```python
from build123d import *

# Parameters (mm, degrees)
RACCORDO1_R              = 1
SMUSSO1_SIZE             = 1
RACCORDO2_R              = 1
TAGLIO_ESTRUSIONE1_DEPTH = 36.80502758


with BuildPart() as part:
    # Schizzo1 → Rivoluzione1 (revolve)
    with BuildSketch(Plane.XY, mode=Mode.PRIVATE) as rivoluzione1_sk:
        Polygon((10.5, 7), (21, 7), (21, 1), (10, 1), (10, 0), (6, 0), (6, 27), (9.5, 27), (9.5, 12), (10.5, 12), align=None)
    revolve(rivoluzione1_sk.sketch.rotate(Axis((0, 27, 0), (0, -1, 0)), 90), axis=Axis((0, 27, 0), (0, -1, 0)))

    # Raccordo1
    raccordo1_edges = [part.edges().sort_by_distance(p)[0] for p in [
        (0, 12, -9.5),
    ]]
    fillet(raccordo1_edges, radius=RACCORDO1_R - 0.0001)  # a hair under: the kernel refuses the full size

    # Smusso1
    smusso1_edges = [part.edges().sort_by_distance(p)[0] for p in [
        (0, 27, -9.5),
    ]]
    chamfer(smusso1_edges, length=SMUSSO1_SIZE)

    # Raccordo2
    raccordo2_edges = [part.edges().sort_by_distance(p)[0] for p in [
        (0, 1, -10),
    ]]
    fillet(raccordo2_edges, radius=RACCORDO2_R - 0.0001)  # a hair under: the kernel refuses the full size

    # Schizzo2 → Taglio-Estrusione1 (cut, through all)
    with BuildSketch(Plane(origin=(0, 7, 0), x_dir=(1, 0, 0), z_dir=(0, 1, 0))):
        with BuildLine():
            ThreePointArc((2.25, 15.5), (1.590990258, 17.090990258), (0, 17.75))
            Line((0, 17.75), (0, 13.25))
            ThreePointArc((0, 13.25), (1.590990258, 13.909009742), (2.25, 15.5))
        make_face()
        with BuildLine():
            Line((0, 13.25), (0, 17.75))
            ThreePointArc((0, 17.75), (-2.25, 15.5), (0, 13.25))
        make_face()
        with BuildLine():
            ThreePointArc((17.75, 0), (15.5, 2.25), (13.25, 0))
            Line((13.25, 0), (17.75, 0))
        make_face()
        with BuildLine():
            Line((17.75, 0), (13.25, 0))
            ThreePointArc((13.25, 0), (15.5, -2.25), (17.75, 0))
        make_face()
        with BuildLine():
            ThreePointArc((2.25, -15.5), (1.590990258, -13.909009742), (0, -13.25))
            Line((0, -13.25), (0, -17.75))
            ThreePointArc((0, -17.75), (1.590990258, -17.090990258), (2.25, -15.5))
        make_face()
        with BuildLine():
            Line((0, -17.75), (0, -13.25))
            ThreePointArc((0, -13.25), (-2.25, -15.5), (0, -17.75))
        make_face()
        with BuildLine():
            ThreePointArc((-17.75, 0), (-15.5, -2.25), (-13.25, 0))
            Line((-13.25, 0), (-17.75, 0))
        make_face()
        with BuildLine():
            Line((-17.75, 0), (-13.25, 0))
            ThreePointArc((-13.25, 0), (-15.5, 2.25), (-17.75, 0))
        make_face()
    extrude(amount=-TAGLIO_ESTRUSIONE1_DEPTH, mode=Mode.SUBTRACT)


solid = part.part
```
Work out the finished part from the listing and answer in its coordinate system (mm). A direction names the side the tool comes from. Give positions to 0.01 mm unless a question says otherwise; leave off trailing zeros. Loops run counter-clockwise (first coordinate to the right, second up) from the corner with the lowest first, then second, coordinate; pieces in that order, holes last. Notation, with made-up numbers: (-36.75, 72) - (-20.75, 72) arc R5 cw to (-20.75, 79) - close; hole circle Ø10 at (-11.5, -36.75). An arc over 180 degrees is marked (long way). One line per question, with ' | ' between items.
(1) A tool of negligible diameter and unlimited length cuts with its end or side. For faces 1 (the face through (-6, 27, -2)), 2 (the face through (-3.2, 9.5, 10)), 3 (the face through (9, 1, 9)), from which of +Z, -Z, +X, -X, +Y, -Y can it reach the whole face along a straight path? Write none if from no direction.
Recorded:
face 1: +Z, -Z, +X, -X, +Y | face 2: +Y | face 3: -Y
(2) The part is cut by section C-C (x = -16). Write down the section's boundary in (y, z).
Recorded:
outline: (1, -13.6) - (7, -13.6) - (7, -2.19) - (1, -2.19) - close; (1, 2.19) - (7, 2.19) - (7, 13.6) - (1, 13.6) - close
(3) The mould has two halves that part along Z. Classify faces 4 (the face through (-1.802, 13.689, 5.723)), 5 (the face through (-10, 7, -4)), 6 (the face through (-6.31, 3.96, 20.03)): +Z half, -Z half, draft (parallel to the pull), parting line (faces both ways), or undercut.
Recorded:
face 4: undercut | face 5: draft | face 6: parting line
(4) Straight lines are drawn through the part: probe 1 along X at (y, z) = (11.75, 0); probe 2 along Y at (x, z) = (-18, 5.5); probe 3 along X at (y, z) = (5.75, 5). For each, find the intervals that lie inside material, in ascending order.
Recorded:
probe 1: x = -10.5 to -6, 6 to 10.5 | probe 2: y = 1 to 7 | probe 3: x = -20.4 to -3.32, 3.32 to 20.4
(5) The part is cut by section D-D (y = 13.75). Write down the section's boundary in (x, z).
Recorded:
outline: circle Ø19 at (0, 0); hole circle Ø12 at (0, 0)
(6) Each of these flat-tipped pins is pushed along its axis until it touches: pin 1 Ø7 at (x, z) = (-15.5, 0) entering from +Y; pin 2 Ø19 at (x, z) = (0, 0) entering from +Y; pin 3 Ø4 at (x, y) = (-0.5, 10) entering from +Z; pin 4 Ø4 at (y, z) = (16.5, -10.5) entering from +X. Where does it stop, or does it pass through?
Recorded:
pin 1: stops at y = 7 | pin 2: stops at y = 27 | pin 3: stops at z = 10.5 | pin 4: stops at x = 4.24
(7) The part is cut by section B-B (z = 0). Count the separate pieces of the cut face and the enclosed holes in it, then the cut area to 3 significant figures.
Recorded:
separate pieces: 4 | enclosed holes: 0 | area: 284 mm²
(8) The part is cut by section A-A (y = 6.25). Write down the section's boundary in (x, z).
Recorded:
outline: circle Ø42 at (0, 0); hole circle Ø4.5 at (-15.5, 0); hole circle Ø12 at (0, 0); hole circle Ø4.5 at (0, -15.5); hole circle Ø4.5 at (0, 15.5); hole circle Ø4.5 at (15.5, 0)
